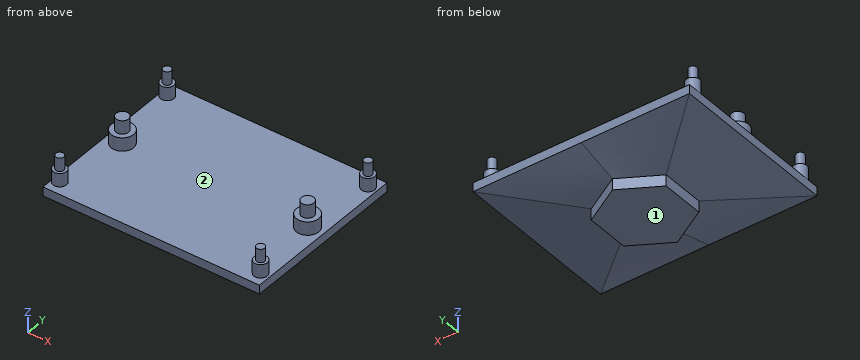
from build123d import *

# Parameters (mm, degrees)
SKIZZE2_2_W                     = 38
SKIZZE2_2_H                     = 48.5
AUFSATZ_LINEAR_AUSTRAGEN1_DEPTH = 2
SKIZZE4_R                       = 2.5
SKIZZE4_R_2                     = 1.5
AUFSATZ_LINEAR_AUSTRAGEN2_DEPTH = 3
SKIZZE5_R                       = 0.9
SKIZZE5_R_2                     = 1.4
AUFSATZ_LINEAR_AUSTRAGEN3_DEPTH = 3


with BuildPart() as part:
    # Skizze1 → Ausformung3 section 0
    with BuildSketch(Plane(origin=(0, 0, 0), x_dir=(0, 1, 0), z_dir=(0, 0, 1))):
        with BuildLine():
            Line((-4.85, 8.400446417), (-9.7, 0))
            Line((-9.7, 0), (-4.85, -8.400446417))
            Line((-4.85, -8.400446417), (4.85, -8.400446417))
            Line((4.85, -8.400446417), (9.7, 0))
            Line((9.7, 0), (4.85, 8.400446417))
            Line((4.85, 8.400446417), (-4.85, 8.400446417))
        make_face()
    # Skizze3 → Ausformung3 section 1
    with BuildSketch(Plane(origin=(0, 0, 2.5), x_dir=(0, 1, 0), z_dir=(0, 0, 1))):
        with BuildLine():
            Line((4.85, 8.400446417), (-4.85, 8.400446417))
            Line((-4.85, 8.400446417), (-9.7, 0))
            Line((-9.7, 0), (-4.85, -8.400446417))
            Line((-4.85, -8.400446417), (4.85, -8.400446417))
            Line((4.85, -8.400446417), (9.7, 0))
            Line((9.7, 0), (4.85, 8.400446417))
        make_face()
    loft()

    # Ausformung4: read off the stored shape, not the designer's step
    # Ausformung4: loft between two sections, ruled curve by curve
    ausformung4_from = [
        Edge.make_bspline([(24.25, -19, 5), (20.208333333, -19, 5), (16.166666667, -19, 5), (8.083333333, -19, 5), (4.041666667, -19, 5), (0, -19, 5)], [0, 0, 0, 0, 0.5, 0.5, 1, 1, 1, 1], 3),
        Edge.make_bspline([(0, -19, 5), (-4.041666667, -19, 5), (-8.083333333, -19, 5), (-16.166666667, -19, 5), (-20.208333333, -19, 5), (-24.25, -19, 5)], [0, 0, 0, 0, 0.5, 0.5, 1, 1, 1, 1], 3),
        Edge.make_bspline([(-24.25, 19, 5), (-20.208333333, 19, 5), (-16.166666667, 19, 5), (-8.083333333, 19, 5), (-4.041666667, 19, 5), (0, 19, 5)], [0, 0, 0, 0, 0.5, 0.5, 1, 1, 1, 1], 3),
        Edge.make_bspline([(0, 19, 5), (4.041666667, 19, 5), (8.083333333, 19, 5), (16.166666667, 19, 5), (20.208333333, 19, 5), (24.25, 19, 5)], [0, 0, 0, 0, 0.5, 0.5, 1, 1, 1, 1], 3),
        Edge.make_line((24.25, -19, 5), (24.25, 19, 5)),
        Edge.make_line((-24.25, 19, 5), (-24.25, -19, 5)),
    ]
    ausformung4_to = [
        Edge.make_bspline([(8.400446417, -4.85, 2.5), (7.000372014, -5.658333333, 2.5), (5.600297611, -6.466666667, 2.5), (2.800148806, -8.083333333, 2.5), (1.400074403, -8.891666667, 2.5), (0, -9.7, 2.5)], [0, 0, 0, 0, 0.5, 0.5, 1, 1, 1, 1], 3),
        Edge.make_bspline([(0, -9.7, 2.5), (-1.400074403, -8.891666667, 2.5), (-2.800148806, -8.083333333, 2.5), (-5.600297611, -6.466666667, 2.5), (-7.000372014, -5.658333333, 2.5), (-8.400446417, -4.85, 2.5)], [0, 0, 0, 0, 0.5, 0.5, 1, 1, 1, 1], 3),
        Edge.make_bspline([(-8.400446417, 4.85, 2.5), (-7.000372014, 5.658333333, 2.5), (-5.600297611, 6.466666667, 2.5), (-2.800148806, 8.083333333, 2.5), (-1.400074403, 8.891666667, 2.5), (0, 9.7, 2.5)], [0, 0, 0, 0, 0.5, 0.5, 1, 1, 1, 1], 3),
        Edge.make_bspline([(0, 9.7, 2.5), (1.400074403, 8.891666667, 2.5), (2.800148806, 8.083333333, 2.5), (5.600297611, 6.466666667, 2.5), (7.000372014, 5.658333333, 2.5), (8.400446417, 4.85, 2.5)], [0, 0, 0, 0, 0.5, 0.5, 1, 1, 1, 1], 3),
        Edge.make_line((8.400446417, -4.85, 2.5), (8.400446417, 4.85, 2.5)),
        Edge.make_line((-8.400446417, 4.85, 2.5), (-8.400446417, -4.85, 2.5)),
    ]
    ausformung4 = Solid(Shell([*[Face.make_surface_from_curves(ausformung4_from[k], ausformung4_to[k]) for k in range(6)], Face(Wire(ausformung4_from)), Face(Wire(ausformung4_to))]))
    add(ausformung4)

    # Skizze2<2> → Aufsatz-Linear austragen1 (add)
    with BuildSketch(Plane(origin=(0, 0, 5), x_dir=(0, 1, 0), z_dir=(0, 0, 1))):
        Rectangle(SKIZZE2_2_W, SKIZZE2_2_H)
    extrude(amount=AUFSATZ_LINEAR_AUSTRAGEN1_DEPTH)

    # Skizze4 → Aufsatz-Linear austragen2 (add)
    with BuildSketch(Plane.XY.offset(7)):
        with Locations((-20.75, 0)):
            Circle(SKIZZE4_R)
        with Locations((20.75, 0)):
            Circle(SKIZZE4_R)
        with Locations(Location((-22.75, 16, 0), (0, 0, 180))):
            Circle(SKIZZE4_R_2)
        with Locations(Location((-22.75, -16, 0), (0, 0, 180))):
            Circle(SKIZZE4_R_2)
        with Locations((22.25, 16)):
            Circle(SKIZZE4_R_2)
        with Locations((22.25, -16)):
            Circle(SKIZZE4_R_2)
    extrude(amount=AUFSATZ_LINEAR_AUSTRAGEN2_DEPTH)

    # Skizze5 → Aufsatz-Linear austragen3 (add)
    with BuildSketch(Plane.XY.offset(10)):
        with Locations((-22.75, 16)):
            Circle(SKIZZE5_R)
        with Locations((-22.75, -16)):
            Circle(SKIZZE5_R)
        with Locations((-20.75, 0)):
            Circle(SKIZZE5_R_2)
        with Locations((20.75, 0)):
            Circle(SKIZZE5_R_2)
        with Locations((22.25, 16)):
            Circle(SKIZZE5_R)
        with Locations((22.25, -16)):
            Circle(SKIZZE5_R)
    extrude(amount=AUFSATZ_LINEAR_AUSTRAGEN3_DEPTH)


solid = part.part
Geometry check sheet. Reference: the model listing, model coordinates, mm. Face numbers are marked on the shaded views. A direction names the side the tool comes from. Round coordinates to 2 decimals unless told otherwise and drop trailing zeros. One line per question, with ' | ' between items. Start each with the question number.
(1) Depth check by flat-ended pin: pin 1 Ø19 at (x, y) = (6.5, 0) entering from +Z; pin 2 Ø5 at (y, z) = (0, 10) entering from +X; pin 3 Ø8 at (x, y) = (-15, -9.5) entering from -Z. Enter the tip coordinate at first touch or a pass-through.
(2) Access from +Z, -Z, +X, -X, +Y, -Y to the whole of each face (thin tool, end or side, straight path). Record for the marked faces 1 and 2.
(3) Thickness scan on L1, parallel to X at y = -3, z = 1.5; L2, parallel to X at y = 2, z = 9; L3, parallel to Z at x = -0.5, y = -9. Record the ranges inside material, lowest first. Write a range as [from, to].
Conclusion:
1) pin 1: stops at z = 7 | pin 2: stops at x = 23.25 | pin 3: stops at z = 2.99
2) face 1: -Z, +X, -X, +Y, -Y | face 2: +Z
3) L1: x = [-8.4, 8.4] | L2: x = [-22.25, -19.25], [19.25, 22.25] | L3: z = [0, 7]
